Job drawing, mm, ordinate dimensions from the low corner. One solid piece. Round coordinates to 2 decimals unless told otherwise and drop trailing zeros. Order: outer loops, then holes, each group sorted by start corner. A loop starts at its lowest first (then second) coordinate and runs counter-clockwise, first axis right, second up. Notation, with made-up numbers: (-4.5, 35) -> (1.5, 35) arc R23 cw to (1.5, 50) -> close; hole circle Ø7 at (9.5, 35.25). An arc over 180 degrees is marked (long way). Write item = value, one per line.
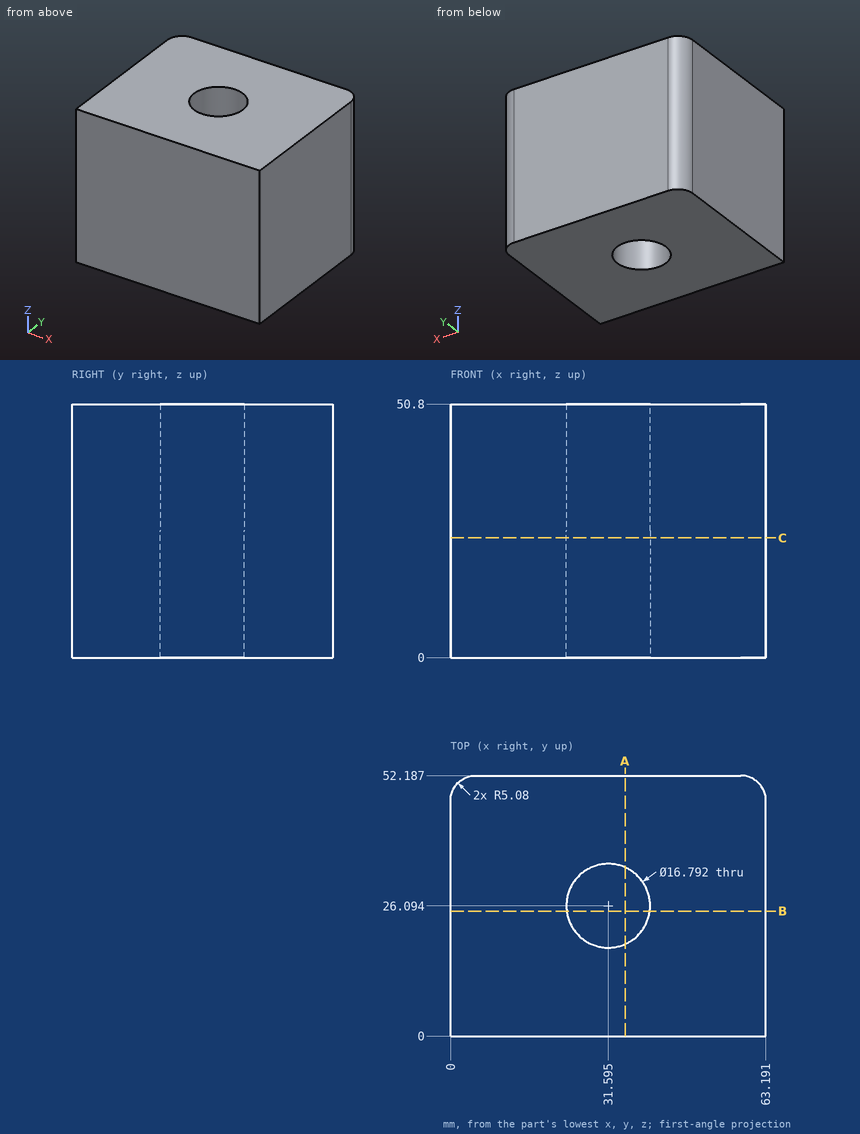
Q1. Probe probe 1 along X at (y, z) = (29.5, 19); probe 2 along X at (y, z) = (25.5, 30); probe 3 along Y at (x, z) = (28.5, 40.5). List the from-to ranges inside material, lowest first.
Check values:
probe_1 = 0 to 23.92, 39.27 to 63.19
probe_2 = 0 to 23.22, 39.97 to 63.19
probe_3 = 0 to 18.29, 33.9 to 52.19
Q2. Cut at C-C, the plane z = 24. List the corners of the cut face in (x, y) (1 decimal), and give its area (4 significant figures).
Check values:
outline = (0, 0) -> (63.2, 0) -> (63.2, 47.1) arc R5.1 ccw to (58.1, 52.2) -> (5.1, 52.2) arc R5.1 ccw to (0, 47.1) -> close; hole circle Ø16.8 at (31.6, 26.1)
area = 3,065 mm²
Q3. Flat gauge pins, fed straight in: pin 1 (13.5 mm diameter, centred on x = 31.6, y = 26.09, fed in from +Z); pin 2 (12 mm diameter, centred on x = 55.5, y = 42.5, fed in from -Z). Where does each tip first touch, or does it go through?
Check values:
pin_1 = through
pin_2 = 0
Q4. Cut at A-A, the plane x = 35. List the corners of the cut face in (y, z), and give its area (3 significant figures).
Check values:
outline = (0, 0) -> (18.42, 0) -> (18.42, 50.8) -> (0, 50.8) -> close; (33.77, 0) -> (52.19, 0) -> (52.19, 50.8) -> (33.77, 50.8) -> close
area = 1,870 mm²
Q5. Cut at B-B, the plane y = 25. List the corners of the cut face in (x, z), and give its area (3 significant figures).
Check values:
outline = (0, 0) -> (23.27, 0) -> (23.27, 50.8) -> (0, 50.8) -> close; (39.92, 0) -> (63.19, 0) -> (63.19, 50.8) -> (39.92, 50.8) -> close
area = 2,360 mm²
